Verification items for the finished model (mm, model axes). A direction names the side the tool comes from. Give positions to 0.01 mm unless a question says otherwise; leave off trailing zeros. Write each loop counter-clockwise with the first axis right and the second up, starting at its lowest first coordinate (ties: lowest second). Pieces come first, ordered by that corner, then holes. Notation, with made-up numbers: (25.5, -2) - (48.5, -2) arc R10 cw to (48.5, 9) - close; hole circle Ø9 at (44, 14). An arc over 180 degrees is marked (long way). Answer as a JSON object with one key per item and string values. Group by question number.
Item 1: Draft check along Z on faces 1 (the face through (0, 19, 351)), 2 (the face through (17.485, 23.246, 100.975)), 3 (the face through (3, 19, 711.2)). Enter one of: +Z half, -Z half, draft (parallel to the pull), parting line (faces both ways), or undercut.
Item 2: Sectioned sample at A-A, the plane y = 19.05. Count the separate pieces of the cut face and the enclosed holes in it, and give its area (3 significant figures).
Item 3: Tool access check on faces 4 (the face through (9, 34.925, 351)), 5 (the face through (1.61, 19.678, 700.074)). Record the directions out of +Z, -Z, +X, -X, +Y, -Y that give a thin tool (end or side, any length) a straight path to the whole face; none if there is none.
Item 4: Sectioned sample at C-C, the plane x = 13. Record the boundary of the cut face in (y, z) (3 decimals), and give its area (3 significant figures).
Item 5: Sectioned sample at D-D, the plane z = 61.5. Record the boundary of the cut face in (x, y) (3 decimals), and give its area (3 significant figures).
Item 6: Scan lines: line 1 along X through (y, z) = (10.5, 380) (3 decimals); line 2 along Y through (x, z) = (17.95, 685.8); line 3 along Y through (x, z) = (15.75, 456) (3 decimals). Record each from-to range of solid material in increasing order. Write a range as [from, to].
```python
from build123d import *

# Parameters (mm, degrees)
SKETCH1_W           = 19.05
SKETCH1_H           = 38.1
SKETCH1_W_2         = 12.7
SKETCH1_H_2         = 31.75
EXTRUDE_THIN1_DEPTH = 711.2
SKETCH3_R           = 13.97
CUT_EXTRUDE2_DEPTH  = 713.474527615
SKETCH4_R           = 14.2875
CUT_EXTRUDE3_DEPTH  = 713.474527615


with BuildPart() as part:
    # Sketch1 → Extrude-Thin1 (new body)
    with BuildSketch(Plane.XY):
        with Locations((9.525, 19.05)):
            Rectangle(SKETCH1_W, SKETCH1_H)
        with Locations((9.525, 19.05)):
            Rectangle(SKETCH1_W_2, SKETCH1_H_2, mode=Mode.SUBTRACT)
    extrude(amount=EXTRUDE_THIN1_DEPTH)

    # Sketch3 → Cut-Extrude2 (cut, through all)
    with BuildSketch(Plane(origin=(19.05, 0, 0), x_dir=(0, 0, -1), z_dir=(1, 0, 0))):
        with Locations((-114.3, 19.05)):
            Circle(SKETCH3_R)
    extrude(amount=-CUT_EXTRUDE2_DEPTH, mode=Mode.SUBTRACT)

    # Sketch4 → Cut-Extrude3 (cut, through all)
    with BuildSketch(Plane(origin=(19.05, 0, 0), x_dir=(0, 0, -1), z_dir=(1, 0, 0))):
        with Locations((-685.8, 19.05)):
            Circle(SKETCH4_R)
    extrude(amount=-CUT_EXTRUDE3_DEPTH, mode=Mode.SUBTRACT)


solid = part.part
```
Geometry check:
{
 "1": {"face 1": "draft", "face 2": "undercut", "face 3": "+Z half"},
 "2": {"separate pieces": "6", "enclosed holes": "0", "area": "4,160 mm^2"},
 "3": {"face 4": "+Z, -Z", "face 5": "+X, -X"},
 "4": {"outline": "(0, 0) - (3.175, 0) - (3.175, 711.2) - (0, 711.2) - close; (34.925, 0) - (38.1, 0) - (38.1, 711.2) - (34.925, 711.2) - close", "area": "4,520 mm^2"},
 "5": {"outline": "(0, 0) - (19.05, 0) - (19.05, 38.1) - (0, 38.1) - close; hole (3.175, 3.175) - (15.875, 3.175) - (15.875, 34.925) - (3.175, 34.925) - close", "area": "323 mm^2"},
 "6": {"line 1": "[0, 3.175], [15.875, 19.05]", "line 2": "[0, 4.76], [33.34, 38.1]", "line 3": "[0, 3.175], [34.925, 38.1]"}
}
